Here's how the part is built. I have some questions about the finished solid (model axes, mm). A direction names the side the tool comes from. Coordinates: 2 decimals unless noted, no trailing zeros. Write each loop counter-clockwise with the first axis right and the second up, starting at its lowest first coordinate (ties: lowest second). Pieces come first, ordered by that corner, then holes. Notation, with made-up numbers: (49.25, -15.75) -> (105.25, -15.75) arc R15 ccw to (105.25, -8.75) -> close; hole circle Ø4 at (70.5, 78). An arc over 180 degrees is marked (long way). Put each result on its own line as item: value. Start each with the question number.
Item 1: If we mould it in two halves opening along Y, with no side actions, what happens to faces 4 (the face through (-0.2, -3.7, 0)), 5 (the face through (8.75, 2.7, 2.47)), 6 (the face through (-8.242, 3.277, 2.465)), 7 (the face through (12, 4.14, 2.46))? For each: released by +Y, released by -Y, zero draft, split by the parting line, or undercut.
Item 2: I want a section at C-C, the plane z = 4. State how many separate pieces and enclosed holes the cut face has, then the cut area to 3 significant figures.
Item 3: For pin 1 (2 mm diameter, centred on x = 10, y = 2.64, fed in from -Z); pin 2 (2.5 mm diameter, centred on x = -12, z = 1.5, fed in from -Y); pin 3 (0.6 mm diameter, centred on y = -2.5, z = 3, fed in from +X); pin 4 (1.5 mm diameter, centred on y = 0.5, z = 1.5, fed in from +X), each with a flat end and sliding along its axis, tell me the tip position at first contact or that it passes through.
Item 4: I want a section at B-B, the plane x = -15.5. List the corners of the cut face in (y, z) for me, then the cut area to 3 significant figures.
Item 5: I want a section at A-A, the plane x = 10. List the corners of the cut face in (y, z) for me.
Item 6: I need wall thicknesses on line 1 (Y direction, x = 10, z = 2.9); line 2 (X direction, y = -3, z = 1.9); line 3 (Y direction, x = -9, z = 1.25). Which ranges of each line are inside material? Lowest first, please. Write a range as [from, to].
Item 7: I want a section at D-D, the plane y = -1.25. List the corners of the cut face in (x, z) for me, then the cut area to 3 significant figures.
Item 8: On a 3-axis mill with a long thin cutter (end or side, diameter ignored), from which of +Z, -Z, +X, -X, +Y, -Y can I reach the whole of each face in a straight line? I mean faces 1 (the face through (0.43, -5.16, 2.54)), 2 (the face through (-11, -5.609, 2)), 3 (the face through (-20, 0.2, 2.5)). Say none if no direction works.
from build123d import *

# Parameters (mm, degrees)
SKETCH1_R           = 1.25
BOSS_EXTRUDE1_DEPTH = 5
FILLET3_R           = 2
FILLET4_R           = 3
FILLET5_R           = 5
FILLET6_R           = 1.5
FILLET8_R           = 0.7
FILLET9_R           = 3


with BuildPart() as part:
    # Sketch1 → Boss-Extrude1 (new body)
    with BuildSketch(Plane.XY):
        with BuildLine():
            Line((10, -0.609130042), (10, 0.141993323))
            ThreePointArc((10, 0.141993323), (11.352749323, 4.744389401), (7.724788103, 1.605937907))
            ThreePointArc((7.724788103, 1.605937907), (-6.192467122, 3.375494669), (-20, 0.890869958))
            Line((-20, 0.890869958), (-20, -0.609130042))
            Line((-20, -0.609130042), (-0.5, -0.609130042))
            Line((-0.5, -0.609130042), (-0.5, -3.109130042))
            Line((-0.5, -3.109130042), (0, -3.109130042))
            Line((0, -3.109130042), (0, -0.609130042))
            Line((0, -0.609130042), (10, -0.609130042))
        make_face()
        with Locations((10, 2.641993323)):
            Circle(SKETCH1_R, mode=Mode.SUBTRACT)
    extrude(amount=BOSS_EXTRUDE1_DEPTH)

    # Fillet3
    fillet3_edges = [part.edges().sort_by_distance(p)[0] for p in [
        (-20, 0.140869958, 0),
        (-20, 0.140869958, 5),
    ]]
    fillet(fillet3_edges, radius=FILLET3_R)

    # Fillet4
    # the kernel refuses this fillet: 3 mm, written as the material it adds along each edge
    with BuildSketch(Plane(origin=(10, 0.141993323, 0), x_dir=(0.9720485785633484, 0.23477981368289305, 0), z_dir=(0, 0, 1))) as fillet4_piece_1:
        with BuildLine():
            CenterArc((1.878238509, -2.916145736), FILLET4_R, 103.578643904, 29.646140471)
            Line((-0.176348604, -0.730128399), (-0.217440346, -0.686408053))
            ThreePointArc((-0.217440346, -0.686408053), (-0.146497217, -0.350977411), (-0.058322915, 0.014086789))
            Line((-0.058322915, 0.014086789), (0.014086789, 0.058322915))
            ThreePointArc((0.014086789, 0.058322915), (0.586949534, -0.009878554), (1.15981228, 0.058322915))
            Line((1.15981228, 0.058322915), (1.173899068, 0))
        make_face()
    extrude(amount=5)

    # Fillet5
    fillet5_edges = [part.edges().sort_by_distance(p)[0] for p in [
        (7.724788103, 1.605937907, 2.5),
    ]]
    fillet(fillet5_edges, radius=FILLET5_R)

    # Mirror2: part across plane


with BuildPart() as part_1:
    add(part.part)
    add(part.part.mirror(Plane(origin=(0, -3.109130042, 0), x_dir=(0, 0, 1), z_dir=(0, -1, 0))))

    # Fillet6
    fillet6_edges = [part_1.edges().sort_by_distance(p)[0] for p in [
        (0, -0.609130042, 2.5),
        (-0.5, -0.609130042, 2.5),
        (-0.5, -5.609130042, 2.5),
        (0, -5.609130042, 2.5),
    ]]
    fillet(fillet6_edges, radius=FILLET6_R)

    # Fillet8
    fillet8_edges = [part_1.edges().sort_by_distance(p)[0] for p in [
        (8.75, 2.641993323, 5),
        (8.75, 2.641993323, 0),
        (8.75, -8.860253407, 5),
        (8.75, -8.860253407, 0),
    ]]
    fillet(fillet8_edges, radius=FILLET8_R)

    # Fillet9
    fillet9_edges = [part_1.edges().sort_by_distance(p)[0] for p in [
        (10, -0.609130042, 2.5),
        (10, -5.609130042, 2.5),
    ]]
    fillet(fillet9_edges, radius=FILLET9_R)


solid = part_1.part
Calculated:
1. face 4: zero draft
1. face 5: undercut
1. face 6: released by +Y
1. face 7: undercut
2. separate pieces: 1
2. enclosed holes: 2
2. area: 226 mm2
3. pin 1: passes through
3. pin 2: stops at y = -9.25
3. pin 3: stops at x = 0
3. pin 4: stops at x = 12.08
4. outline: (-8.4, 0) -> (-5.61, 0) -> (-5.61, 5) -> (-8.4, 5) -> close; (-0.61, 0) -> (2.18, 0) -> (2.18, 5) -> (-0.61, 5) -> close
4. area: 27.9 mm2
5. outline: (-11.36, 0) -> (-10.81, 0) arc R0.7 ccw to (-10.11, 0.7) -> (-10.11, 4.3) arc R0.7 ccw to (-10.81, 5) -> (-11.36, 5) -> close; (-7.61, 0.7) arc R0.7 ccw to (-6.91, 0) -> (-5.9, 0) -> (-5.9, 5) -> (-6.91, 5) arc R0.7 ccw to (-7.61, 4.3) -> close; (-0.32, 0) -> (0.69, 0) arc R0.7 ccw to (1.39, 0.7) -> (1.39, 4.3) arc R0.7 ccw to (0.69, 5) -> (-0.32, 5) -> close; (3.89, 0.7) arc R0.7 ccw to (4.59, 0) -> (5.14, 0) -> (5.14, 5) -> (4.59, 5) arc R0.7 ccw to (3.89, 4.3) -> close
6. line 1: y = [-11.36, -10.11], [-7.61, -5.9], [-0.32, 1.39], [3.89, 5.14]
6. line 2: x = [-0.5, 0]
6. line 3: y = [-9.44, -5.61], [-0.61, 3.22]
7. outline: (-0.77, 0) -> (0.27, 0) -> (0.27, 5) -> (-0.77, 5) -> close
7. area: 5.20 mm2
8. face 1: +Z, -Z, +X
8. face 2: +Z, -Z, -X
8. face 3: +Z, -Z, -X, +Y, -Y
